Here's how the part is built. I have some questions about the finished solid (model axes, mm). Face numbers are marked on the shaded views. A direction names the side the tool comes from. Round coordinates to 2 decimals unless told otherwise and drop trailing zeros. Order: outer loops, then holes, each group sorted by start corner. A loop starts at its lowest first (then second) coordinate and runs counter-clockwise, first axis right, second up. Notation, with made-up numbers: (13.5, 79) -> (72.5, 79) arc R32 cw to (72.5, 105) -> close; hole circle Ø10 at (-36.75, -20.75). An arc over 180 degrees is marked (long way). Use a Markdown table: item, result. Add a question column.
from build123d import *

# Parameters (mm, degrees)
SKETCH1_W                                         = 91
SKETCH1_H                                         = 70
BOSS_EXTRUDE1_DEPTH                               = 9
BOSS_EXTRUDE2_DEPTH                               = 31
SKETCH3_W                                         = 5.6
SKETCH3_H                                         = 10.5
CUT_EXTRUDE1_DEPTH                                = 31
SKETCH4_W                                         = 4.7
SKETCH4_H                                         = 4.9
BOSS_EXTRUDE3_DEPTH                               = 18.5
FILLET1_R                                         = 2
SKETCH5_W                                         = 1.9
SKETCH5_H                                         = 5.8
CUT_EXTRUDE2_DEPTH                                = 19
CSK_FOR_M3_5_FLAT_HEAD_MACHINE_SCREW1_D           = 4.2
CSK_FOR_M3_5_FLAT_HEAD_MACHINE_SCREW1_CSINK_D     = 8.2
CSK_FOR_M3_5_FLAT_HEAD_MACHINE_SCREW1_CSINK_ANGLE = 90
SKETCH11_W                                        = 101.27142764
SKETCH11_H                                        = 82.667879483
SKETCH11_W_2                                      = 85
SKETCH11_H_2                                      = 73.983129472
CUT_EXTRUDE4_DEPTH                                = 49
SKETCH12_W                                        = 32
SKETCH12_H                                        = 15
CUT_EXTRUDE5_DEPTH                                = 5.5
FILLET3_R                                         = 15
FILLET3_OF_MIRROR1_R                              = 15
SKETCH13_W                                        = 85
SKETCH13_H                                        = 10
CUT_EXTRUDE6_DEPTH                                = 53
SKETCH14_W                                        = 23
SKETCH14_H                                        = 31
CUT_EXTRUDE7_DEPTH                                = 10


with BuildPart() as part:
    # Sketch1 → Boss-Extrude1 (new body)
    with BuildSketch(Plane(origin=(0, 0, 0), x_dir=(1, 0, 0), z_dir=(0, 1, 0))):
        Rectangle(SKETCH1_W, SKETCH1_H)
    extrude(amount=BOSS_EXTRUDE1_DEPTH)

    # Sketch2 → Boss-Extrude2 (add)
    with BuildSketch(Plane(origin=(0, 9, 0), x_dir=(1, 0, 0), z_dir=(0, 1, 0))):
        Polygon((-33.5, -35), (-33.5, 28), (33.5, 28), (33.5, -35), (45.5, -35), (45.5, 35), (-45.5, 35), (-45.5, -35), align=None)
    extrude(amount=BOSS_EXTRUDE2_DEPTH)

    # Sketch3 → Cut-Extrude1 (cut)
    with BuildSketch(Plane(origin=(0, 40, 0), x_dir=(1, 0, 0), z_dir=(0, 1, 0))):
        with Locations((-36.3, -15.95)):
            Rectangle(SKETCH3_W, SKETCH3_H)
        with Locations((36.3, -15.95)):
            Rectangle(SKETCH3_W, SKETCH3_H)
    extrude(amount=-CUT_EXTRUDE1_DEPTH, mode=Mode.SUBTRACT)

    # Sketch4 → Boss-Extrude3 (add)
    with BuildSketch(Plane(origin=(0, 9, 0), x_dir=(1, 0, 0), z_dir=(0, 1, 0))):
        with Locations((-7.15, 25.55)):
            Rectangle(SKETCH4_W, SKETCH4_H)
        with Locations((7.15, 25.55)):
            Rectangle(SKETCH4_W, SKETCH4_H)
    extrude(amount=BOSS_EXTRUDE3_DEPTH)

    # Fillet1
    fillet1_edges = [part.edges().sort_by_distance(p)[0] for p in [
        (-9.5, 27.5, -25.55),
        (-4.8, 27.5, -25.55),
        (4.8, 27.5, -25.55),
        (9.5, 27.5, -25.55),
    ]]
    fillet(fillet1_edges, radius=FILLET1_R)

    # Sketch5 → Cut-Extrude2 (cut)
    with BuildSketch(Plane(origin=(0, 9, 0), x_dir=(1, 0, 0), z_dir=(0, 1, 0))):
        with Locations((-19.05, 10.1)):
            Rectangle(SKETCH5_W, SKETCH5_H)
        with Locations((6.55, 10.1)):
            Rectangle(SKETCH5_W, SKETCH5_H)
    extrude(amount=-CUT_EXTRUDE2_DEPTH, mode=Mode.SUBTRACT)

    # CSK for M3.5 Flat Head Machine Screw1 (through all)
    with Locations(Plane(origin=(-20.5, 9, 6), x_dir=(0, 0, 1), z_dir=(0, 1, 0))):
        with Locations((0, 0), (0, 41)):
            CounterSinkHole(CSK_FOR_M3_5_FLAT_HEAD_MACHINE_SCREW1_D / 2, CSK_FOR_M3_5_FLAT_HEAD_MACHINE_SCREW1_CSINK_D / 2, counter_sink_angle=CSK_FOR_M3_5_FLAT_HEAD_MACHINE_SCREW1_CSINK_ANGLE)

    # Sketch11 → Cut-Extrude4 (cut)
    with BuildSketch(Plane(origin=(0, 40, 0), x_dir=(1, 0, 0), z_dir=(0, 1, 0))):
        with Locations((-0.171320914, -3.126256715)):
            Rectangle(SKETCH11_W, SKETCH11_H)
        with Locations((0, -3.991564736)):
            Rectangle(SKETCH11_W_2, SKETCH11_H_2, mode=Mode.SUBTRACT)
    extrude(amount=-CUT_EXTRUDE4_DEPTH, mode=Mode.SUBTRACT)

    # Sketch12 → Cut-Extrude5 (cut)
    with BuildSketch(Plane.ZY.offset(42.5)):
        with Locations((-7, 20)):
            Rectangle(SKETCH12_W, SKETCH12_H)
    cut_extrude5 = extrude(amount=-CUT_EXTRUDE5_DEPTH, mode=Mode.SUBTRACT)

    # Fillet3
    # the kernel refuses this fillet: 15 mm, written as the material it adds along each edge
    with BuildSketch(Plane(origin=(-37, 27.5, 9), x_dir=(-1, 0, 0), z_dir=(0, -1, 0))) as fillet3_piece_1:
        with BuildLine():
            CenterArc((15, 11.608186766), FILLET3_R, 180, 50.703519761)
            Line((0, 11.608186766), (-0.3, 11.608186766))
            Line((-0.3, 11.608186766), (-0.3, 0))
            Line((-0.3, 0), (0, -0.3))
            ThreePointArc((0, -0.3), (2.75, -0.3), (5.31, -0.232163735))
            Line((5.31, -0.232163735), (5.5, 0))
        make_face()
    extrude(amount=15)

    # Mirror1: Cut-Extrude5 across plane
    add(cut_extrude5.mirror(Plane(origin=(0, 0, 0), x_dir=(0, 0, 1), z_dir=(1, 0, 0))), mode=Mode.SUBTRACT)

    # Fillet3 of Mirror1
    # the kernel refuses this fillet: 15 mm, written as the material it adds along each edge
    with BuildSketch(Plane(origin=(37, 27.5, 9), x_dir=(1, 0, 0), z_dir=(0, -1, 0))) as fillet3_of_mirror1_piece_1:
        with BuildLine():
            CenterArc((15, -11.608186766), FILLET3_OF_MIRROR1_R, 129.296480239, 50.703519761)
            Line((0, -11.608186766), (-0.3, -11.608186766))
            Line((-0.3, -11.608186766), (-0.3, 0))
            Line((-0.3, 0), (0, 0.3))
            ThreePointArc((0, 0.3), (2.75, 0.3), (5.31, 0.232163735))
            Line((5.31, 0.232163735), (5.5, 0))
        make_face()
    extrude(amount=15)

    # Sketch13 → Cut-Extrude6 (cut)
    with BuildSketch(Plane(origin=(0, 40, 0), x_dir=(1, 0, 0), z_dir=(0, 1, 0))):
        with Locations((0, -30)):
            Rectangle(SKETCH13_W, SKETCH13_H)
    extrude(amount=-CUT_EXTRUDE6_DEPTH, mode=Mode.SUBTRACT)

    # Sketch14 → Cut-Extrude7 (cut)
    with BuildSketch(Plane.XY.offset(-28)):
        with Locations((-1.5, 24.5)):
            Rectangle(SKETCH14_W, SKETCH14_H)
    extrude(amount=CUT_EXTRUDE7_DEPTH, mode=Mode.SUBTRACT)


solid = part.part
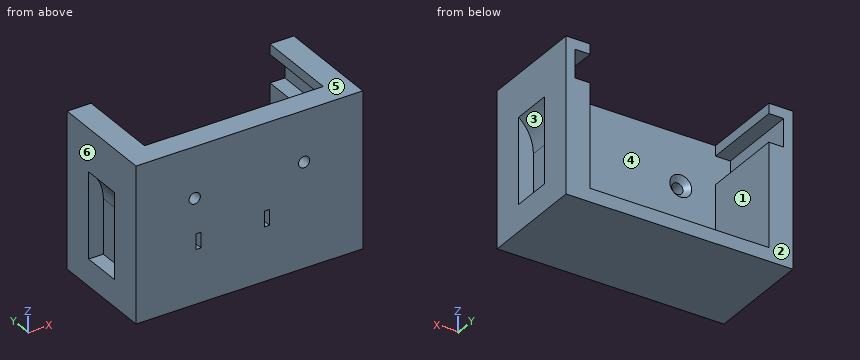
(1) I want a section at B-B on y = 23.5. List the corners of the cut face in (x, z) for me, and give its area (3 significant figures).
(2) I want a section at A-A on z = 19.5. List the corners of the cut face in (x, y) for me, and give its area (3 significant figures).
(3) Please list where these lines run through material, in increasing order: probe 1 along X at (y, z) = (3, 6); probe 2 along X at (y, z) = (36, -8); probe 3 along Y at (x, z) = (38.5, -4.5). Write a range as from..to.
(4) I want a section at D-D on z = 6. List the corners of the cut face in (x, y) for me, and give its area (3 significant figures).
(5) I want a section at C-C on x = 20.5. List the corners of the cut face in (y, z) for me.
(6) On a 3-axis mill with a long thin cutter (end or side, diameter ignored), from which of +Z, -Z, +X, -X, +Y, -Y can I reach the whole of each face in a straight line? I mean the marked faces 1, 2 and 3. Say none if no direction works.
(7) I'm going to push flat-ended pins straight in: P1, Ø12, axis at y = 16.5, z = -9, coming from the -X side; P2, Ø2, axis at y = 18.5, z = -10.5, coming from the -X side; P3, Ø6, axis at x = 15, z = 17.5, coming from the +Y side. Where does each tip first touch, or does it pass through?
(8) If we mould it in two halves opening along X, with no side actions, what happens to the marked faces 4, 5 and 6? For each: pulls with the +X half, pulls with the -X half, needs draft (parallel to the pull), parting line crosses it, or undercut.
Output:
| question | item | result |
|---|---|---|
| 1 | outline | (-42.5, -33) -> (42.5, -33) -> (42.5, -23) -> (37, -23) -> (37, -2.61) arc R15 cw to (42.5, 9) -> (42.5, 25) -> (33.5, 25) -> (33.5, 21.2) -> (39.1, 21.2) -> (39.1, 10.7) -> (33.5, 10.7) -> (33.5, -28) -> (-33.5, -28) -> (-33.5, 10.7) -> (-39.1, 10.7) -> (-39.1, 21.2) -> (-33.5, 21.2) -> (-33.5, 25) -> (-42.5, 25) -> (-42.5, 9) arc R15 cw to (-37, -2.61) -> (-37, -23) -> (-42.5, -23) -> close |
| 1 | area | 948 mm² |
| 2 | outline | (-42.5, 0) -> (42.5, 0) -> (42.5, 40) -> (39.1, 40) -> (39.1, 9) -> (-39.1, 9) -> (-39.1, 40) -> (-42.5, 40) -> close |
| 2 | area | 976 mm² |
| 3 | probe 1 | -42.5..-22.6, -18.4..18.4, 22.6..42.5 |
| 3 | probe 2 | -42.5..-33.5, 33.5..42.5 |
| 3 | probe 3 | 0..12.5, 27.5..40 |
| 4 | outline | (-42.5, 0) -> (-22.6, 0) -> (-22.6, 7) -> (-24.6, 9) -> (-33.5, 9) -> (-33.5, 40) -> (-42.5, 40) -> (-42.5, 27.5) -> (-39.72, 27.5) -> (-39.72, 12.5) -> (-42.5, 12.5) -> close; (-18.4, 0) -> (18.4, 0) -> (18.4, 7) -> (16.4, 9) -> (-16.4, 9) -> (-18.4, 7) -> close; (22.6, 0) -> (42.5, 0) -> (42.5, 12.5) -> (39.72, 12.5) -> (39.72, 27.5) -> (42.5, 27.5) -> (42.5, 40) -> (33.5, 40) -> (33.5, 9) -> (24.6, 9) -> (22.6, 7) -> close |
| 4 | area | 1,160 mm² |
| 5 | outline | (0, -33) -> (40, -33) -> (40, -28) -> (9, -28) -> (9, 1.9) -> (7, 3.9) -> (0, 3.9) -> close; (0, 8.1) -> (7, 8.1) -> (9, 10.1) -> (9, 25) -> (0, 25) -> close |
| 6 | face 1 | +Z, +Y |
| 6 | face 2 | +Z, -Z, +X, -X, +Y |
| 6 | face 3 | +X |
| 7 | P1 | x = -42.5 |
| 7 | P2 | x = -37 |
| 7 | P3 | y = 9 |
| 8 | face 4 | undercut |
| 8 | face 5 | needs draft |
| 8 | face 6 | pulls with the -X half |
